from build123d import *

# Parameters (mm, degrees)
BOSS_EXTRUDE1_DEPTH = 1.524


with BuildPart() as part:
    # Sketch1 → Boss-Extrude1 (new body)
    with BuildSketch(Plane.XY):
        with BuildLine():
            Line((7.568674397, 15.582558464), (-5.536256919, 4.066414385))
            Line((-5.536256919, 4.066414385), (-6.530313076, 5.198282058))
            Line((-6.530313076, 5.198282058), (5.556223507, 15.819133016))
            ThreePointArc((5.556223507, 15.819133016), (5.777089873, 16.550462951), (5.218621489, 17.071748372))
            ThreePointArc((5.218621489, 17.071748372), (3.288269389, 17.169456569), (1.409525645, 16.715443282))
            ThreePointArc((1.409525645, 16.715443282), (1.003306116, 16.541109193), (0.599038273, 16.362295908))
            ThreePointArc((0.599038273, 16.362295908), (-2.550127925, 16.078915888), (-5.536256919, 15.03940369))
            ThreePointArc((-5.536256919, 15.03940369), (-4.380758941, 14.936898454), (-3.431369122, 14.270308722))
            ThreePointArc((-3.431369122, 14.270308722), (-5.61253751, 12.87862193), (-7.699155785, 11.348814153))
            ThreePointArc((-7.699155785, 11.348814153), (-10.424357394, 10.705874365), (-12.591632165, 8.933019197))
            ThreePointArc((-12.591632165, 8.933019197), (-11.673431217, 9.06564735), (-10.902633402, 8.549358731))
            ThreePointArc((-10.902633402, 8.549358731), (-13.90878858, 5.282464583), (-16.534336918, 1.702511755))
            ThreePointArc((-16.534336918, 1.702511755), (-18.59519403, 0.456840392), (-20.068993111, -1.447561206))
            ThreePointArc((-20.068993111, -1.447561206), (-19.197525413, -1.237616175), (-18.302618639, -1.289333967))
            ThreePointArc((-18.302618639, -1.289333967), (-18.746738742, -2.146015126), (-19.170061319, -3.013161751))
            ThreePointArc((-19.170061319, -3.013161751), (-20.151793191, -6.776607347), (-19.40772228, -10.594156129))
            ThreePointArc((-19.40772228, -10.594156129), (-20.160576804, -10.75613538), (-20.886030658, -10.497786933))
            ThreePointArc((-20.886030658, -10.497786933), (-19.40772228, -12.558219915), (-17.161873617, -13.735905577))
            ThreePointArc((-17.161873617, -13.735905577), (-14.272607306, -16.011724419), (-10.902633402, -17.484981731))
            ThreePointArc((-10.902633402, -17.484981731), (-11.686238888, -17.939086495), (-12.591632165, -17.961707434))
            ThreePointArc((-12.591632165, -17.961707434), (-8.881936241, -18.592642939), (-5.172240316, -17.961707434))
            ThreePointArc((-5.172240316, -17.961707434), (-3.516074533, -17.724342682), (-1.880821012, -17.370544649))
            ThreePointArc((-1.880821012, -17.370544649), (-1.897285647, -18.401111131), (-2.412003394, -19.294085934))
            ThreePointArc((-2.412003394, -19.294085934), (0.557596733, -17.882208081), (2.910422529, -15.585224243))
            ThreePointArc((2.910422529, -15.585224243), (6.522466187, -13.346484728), (9.675834999, -10.497786933))
            ThreePointArc((9.675834999, -10.497786933), (9.916567514, -11.124520652), (9.960567596, -11.794454448))
            ThreePointArc((9.960567596, -11.794454448), (10.971969999, -10.129349123), (11.507200123, -8.256106139))
            ThreePointArc((11.507200123, -8.256106139), (12.962197209, -5.968399457), (14.145957127, -3.529274442))
            ThreePointArc((14.145957127, -3.529274442), (14.491523151, -3.864332581), (14.749497984, -4.270693035))
            ThreePointArc((14.749497984, -4.270693035), (15.035659281, -2.627123404), (15.04635356, -0.958862317))
            ThreePointArc((15.04635356, -0.958862317), (15.654704723, 1.754409987), (15.940567857, 4.520313094))
            ThreePointArc((15.940567857, 4.520313094), (16.377113792, 4.256299615), (16.690299619, 3.853571284))
            ThreePointArc((16.690299619, 3.853571284), (16.588539506, 5.261834916), (15.944497262, 6.518326526))
            ThreePointArc((15.944497262, 6.518326526), (14.706822394, 10.090010141), (16.56074466, 13.384207335))
            Line((16.56074466, 13.384207335), (24.140280678, 18.409177712))
            ThreePointArc((24.140280678, 18.409177712), (17.01748918, 17.916684767), (10.115138619, 16.090687846))
            ThreePointArc((10.115138619, 16.090687846), (9.22182641, 15.690950119), (8.244138062, 15.734795847))
            ThreePointArc((8.244138062, 15.734795847), (7.886999128, 15.744784733), (7.568674397, 15.582558464))
        make_face()
    extrude(amount=BOSS_EXTRUDE1_DEPTH)


solid = part.part
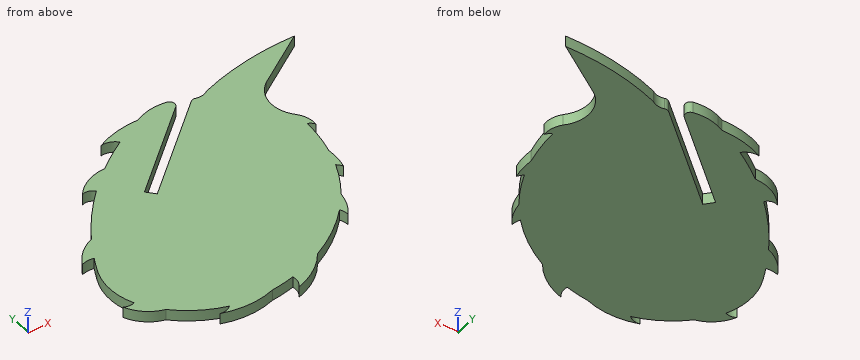
Can you work these out from the model? Positions are in its coordinate system, mm. Give positions to 0.01 mm unless a question says otherwise; leave off trailing zeros. Write each loop counter-clockwise with the first axis right and the second up, starting at its lowest first coordinate (ties: lowest second). Pieces come first, ordered by that corner, then holes. Notation, with made-up numbers: (49.5, -35) -> (71.5, -35) arc R19 ccw to (71.5, -2) -> close; hole circle Ø10 at (8.25, 66). An arc over 180 degrees is marked (long way). Answer as a JSON object with one key per item and string values. Group by question number.
Item 1: Suppose I cut it at C-C (x = 13). Please give me the cut outline in (y, z) (3 decimals), plus the area to 3 significant figures.
Item 2: Suppose I cut it at D-D (x = 19.5). Please give me the cut outline in (y, z).
Item 3: Suppose I cut it at A-A (y = 8). Please give me the cut outline in (x, z).
Item 4: Please list where these lines run through material, in increasing order: line 1 (Y direction, x = -4.5, z = 1.45); line 2 (X direction, y = -4, z = 0.2); line 3 (Y direction, x = 0, z = 1.15). Write a range as [from, to].
Item 5: Suppose I cut it at B-B (x = 4). Please give me the cut outline in (y, z).
Findings:
{
 "1": {"outline": "(-5.9, 0) -> (17.025, 0) -> (17.025, 1.524) -> (-5.9, 1.524) -> close", "area": "34.9 mm²"},
 "2": {"outline": "(15.33, 0) -> (18.24, 0) -> (18.24, 1.52) -> (15.33, 1.52) -> close"},
 "3": {"outline": "(-11.46, 0) -> (-3.34, 0) -> (-3.34, 1.52) -> (-11.46, 1.52) -> close; (-1.06, 0) -> (15.01, 0) -> (15.01, 1.52) -> (-1.06, 1.52) -> close"},
 "4": {"line 1": "y = [-17.88, 4.98], [6.98, 13.61], [14.98, 15.49]", "line 2": "x = [-19.61, 13.94], [14.59, 14.82]", "line 3": "y = [-18.24, 8.93], [10.94, 16.37]"},
 "5": {"outline": "(-15, 0) -> (12.45, 0) -> (12.45, 1.52) -> (-15, 1.52) -> close; (14.45, 0) -> (17.2, 0) -> (17.2, 1.52) -> (14.45, 1.52) -> close"}
}
